from build123d import *

# Parameters (mm, degrees)
SKETCH1_R           = 3.96875
SKETCH1_R_2         = 3.175
BOSS_EXTRUDE1_DEPTH = 5.08
FILLET1_R           = 2.54


with BuildPart() as part:
    # Sketch1 → Boss-Extrude1 (new body)
    with BuildSketch(Plane.XY):
        with BuildLine():
            Line((-11.1125, 15.6083), (-11.1125, 12.7))
            Line((-11.1125, 12.7), (-11.1125, -12.7))
            Line((-11.1125, -12.7), (11.1125, -12.7))
            Line((11.1125, -12.7), (11.1125, 12.7))
            Line((11.1125, 12.7), (11.1125, 15.6083))
            ThreePointArc((11.1125, 15.6083), (0, 26.7208), (-11.1125, 15.6083))
        make_face()
        with Locations((0, 15.6083)):
            Circle(SKETCH1_R, mode=Mode.SUBTRACT)
        with Locations((-5.55625, 0)):
            Circle(SKETCH1_R_2, mode=Mode.SUBTRACT)
        with Locations((5.55625, 0)):
            Circle(SKETCH1_R_2, mode=Mode.SUBTRACT)
    extrude(amount=BOSS_EXTRUDE1_DEPTH)

    # Fillet1
    fillet1_edges = [part.edges().sort_by_distance(p)[0] for p in [
        (11.1125, -12.7, 2.54),
        (-11.1125, -12.7, 2.54),
    ]]
    fillet(fillet1_edges, radius=FILLET1_R)


solid = part.part
Here's how the part is built. I have some questions about the finished solid (model axes, mm). Give positions to 0.01 mm unless a question says otherwise; leave off trailing zeros. Loops run counter-clockwise (first coordinate to the right, second up) from the corner with the lowest first, then second, coordinate; pieces in that order, holes last. Notation, with made-up numbers: (51.5, -39) -> (78.5, -39) arc R31 cw to (78.5, -11) -> close; hole circle Ø4 at (63, 67). An arc over 180 degrees is marked (long way). Answer as a JSON object with one key per item and string values. Group by question number.
Item 1: I need wall thicknesses on L1, parallel to X at y = 15.5, z = 3.3; L2, parallel to Y at x = 0, z = 3.2; L3, parallel to X at y = 19, z = 4.8. Which ranges of each line are inside material? Lowest first, please.
Item 2: Imagine slicing it at B-B on x = 0. Write out the boundary of the cut face in (y, z), then the cut area to 3 significant figures.
Item 3: Imagine slicing it at A-A on y = 0. Write out the boundary of the cut face in (x, z).
Item 4: Imagine slicing it at C-C on z = 2.35. Give the number of separate pieces and of enclosed holes in the cut face, then the cut area to 3 significant figures.
Item 5: Will these pins go through, and if not, where does the flat tip stop? pin 1 (7 mm diameter, centred on x = 0, y = 15.61, fed in from +Z); pin 2 (1.5 mm diameter, centred on y = 21, z = 0.5, fed in from -X).
Item 6: Thinking about a two-plate mould opening in Y: for faces 1 (the flat face through (0, 7, 0)), 2 (the cylindrical face through (7.021, -2.817, 2.504)), 3 (the cylindrical face through (10.349, -11.976, 2.576)), 4 (the cylindrical face through (-0.517, 19.543, 2.504)), which applies, pulls with the +Y half, pulls with the -Y half, needs draft (parallel to the pull), parting line crosses it, or undercut?
Item 7: Imagine slicing it at D-D on y = 15. Write out the boundary of the cut face in (x, z), then the cut area to 3 significant figures.
Answer list:
{
 "1": {"L1": "x = -11.11 to -3.97, 3.97 to 11.11", "L2": "y = -12.7 to 11.64, 19.58 to 26.72", "L3": "x = -10.58 to -2.06, 2.06 to 10.58"},
 "2": {"outline": "(-12.7, 0) -> (11.64, 0) -> (11.64, 5.08) -> (-12.7, 5.08) -> close; (19.58, 0) -> (26.72, 0) -> (26.72, 5.08) -> (19.58, 5.08) -> close", "area": "160 mm2"},
 "3": {"outline": "(-11.11, 0) -> (-8.73, 0) -> (-8.73, 5.08) -> (-11.11, 5.08) -> close; (-2.38, 0) -> (2.38, 0) -> (2.38, 5.08) -> (-2.38, 5.08) -> close; (8.73, 0) -> (11.11, 0) -> (11.11, 5.08) -> (8.73, 5.08) -> close"},
 "4": {"separate pieces": "1", "enclosed holes": "3", "area": "708 mm2"},
 "5": {"pin 1": "passes through", "pin 2": "stops at x = -10.1"},
 "6": {"face 1": "needs draft", "face 2": "undercut", "face 3": "pulls with the -Y half", "face 4": "undercut"},
 "7": {"outline": "(-11.11, 0) -> (-3.92, 0) -> (-3.92, 5.08) -> (-11.11, 5.08) -> close; (3.92, 0) -> (11.11, 0) -> (11.11, 5.08) -> (3.92, 5.08) -> close", "area": "73.1 mm2"}
}
